from build123d import *

# Parameters (mm, degrees)
F0_R     = 5.25
F0_R_2   = 18.800913
F0_R_3   = 5.254085
F0_R_4   = 5.311104
F1_DEPTH = 10


with BuildPart() as f1:
    # F0 (on Front) → F1 (new body)
    with BuildSketch(Plane.XZ):
        with BuildLine():
            Line((195, 23.072333), (195, 73.480297))
            ThreePointArc((195, 73.480297), (193.122359, 78.251192), (188.496733, 80.46265))
            Line((188.496733, 80.46265), (185.082949, 80.705511))
            ThreePointArc((185.082949, 80.705511), (180.133201, 78.655259), (178.082949, 73.705511))
            Line((178.082949, 73.705511), (178.082949, 72.705511))
            ThreePointArc((178.082949, 72.705511), (176.032696, 67.755764), (171.082949, 65.705511))
            Line((171.082949, 65.705511), (110.082949, 65.705511))
            ThreePointArc((110.082949, 65.705511), (105.133201, 67.755764), (103.082949, 72.705511))
            Line((103.082949, 72.705511), (103.082949, 73.705511))
            ThreePointArc((103.082949, 73.705511), (101.032696, 78.655259), (96.082949, 80.705511))
            Line((96.082949, 80.705511), (93.082949, 80.705511))
            ThreePointArc((93.082949, 80.705511), (88.133201, 78.655259), (86.082949, 73.705511))
            Line((86.082949, 73.705511), (86.082949, 72.705511))
            ThreePointArc((86.082949, 72.705511), (84.032696, 67.755764), (79.082949, 65.705511))
            Line((79.082949, 65.705511), (18.082949, 65.705511))
            ThreePointArc((18.082949, 65.705511), (13.133201, 67.755764), (11.082949, 72.705511))
            Line((11.082949, 72.705511), (11.082949, 73.705511))
            ThreePointArc((11.082949, 73.705511), (9.032696, 78.655259), (4.082949, 80.705511))
            Line((4.082949, 80.705511), (1.082949, 80.705511))
            ThreePointArc((1.082949, 80.705511), (-3.866799, 78.655259), (-5.917051, 73.705511))
            Line((-5.917051, 73.705511), (-5.917051, 72.705511))
            ThreePointArc((-5.917051, 72.705511), (-7.967304, 67.755764), (-12.917051, 65.705511))
            Line((-12.917051, 65.705511), (-73.917051, 65.705511))
            ThreePointArc((-73.917051, 65.705511), (-78.866799, 67.755764), (-80.917051, 72.705511))
            Line((-80.917051, 72.705511), (-80.917051, 73.705511))
            ThreePointArc((-80.917051, 73.705511), (-82.967304, 78.655259), (-87.917051, 80.705511))
            Line((-87.917051, 80.705511), (-90.917051, 80.705511))
            ThreePointArc((-90.917051, 80.705511), (-95.866799, 78.655259), (-97.917051, 73.705511))
            Line((-97.917051, 73.705511), (-97.917051, 72.705511))
            ThreePointArc((-97.917051, 72.705511), (-99.967304, 67.755764), (-104.917051, 65.705511))
            Line((-104.917051, 65.705511), (-165.917051, 65.705511))
            ThreePointArc((-165.917051, 65.705511), (-170.866799, 67.755764), (-172.917051, 72.705511))
            Line((-172.917051, 72.705511), (-172.917051, 73.705511))
            ThreePointArc((-172.917051, 73.705511), (-174.967304, 78.655259), (-179.917051, 80.705511))
            Line((-179.917051, 80.705511), (-187.917051, 80.705511))
            ThreePointArc((-187.917051, 80.705511), (-191.62203, 79.64463), (-194.203996, 76.78355))
            ThreePointArc((-194.203996, 76.78355), (-194.606342, 74.960742), (-194.128551, 73.156241))
            Line((-194.128551, 73.156241), (-190.179633, 51.218559))
            ThreePointArc((-190.179633, 51.218559), (-190.114418, 50.911785), (-190.030097, 50.609704))
            Line((-190.030097, 50.609704), (-186.59138, 39.632266))
            ThreePointArc((-186.59138, 39.632266), (-186.208592, 38.609697), (-185.716602, 37.634957))
            Line((-185.716602, 37.634957), (-177.611824, 23.546821))
            ThreePointArc((-177.611824, 23.546821), (-176.740115, 22.270978), (-175.682257, 21.144661))
            Line((-175.682257, 21.144661), (-171.066362, 16.935058))
            ThreePointArc((-171.066362, 16.935058), (-169.380238, 14.933988), (-168.270966, 12.564006))
            Line((-168.270966, 12.564006), (-165.841167, 4.887599))
            ThreePointArc((-165.841167, 4.887599), (-163.303518, 1.352575), (-159.167506, 0))
            Line((-159.167506, 0), (-155, 0))
            Line((-155, 0), (-150.832494, 0))
            ThreePointArc((-150.832494, 0), (-146.696482, 1.352575), (-144.158833, 4.887599))
            Line((-144.158833, 4.887599), (-141.729034, 12.564006))
            ThreePointArc((-141.729034, 12.564006), (-140.619762, 14.933988), (-138.933638, 16.935058))
            Line((-138.933638, 16.935058), (-134.317743, 21.144661))
            ThreePointArc((-134.317743, 21.144661), (-133.259885, 22.270978), (-132.388176, 23.546821))
            Line((-132.388176, 23.546821), (-124.283398, 37.634957))
            Line((-124.283398, 37.634957), (-95.716602, 37.634957))
            Line((-95.716602, 37.634957), (-87.611824, 23.546821))
            ThreePointArc((-87.611824, 23.546821), (-86.740115, 22.270978), (-85.682257, 21.144661))
            Line((-85.682257, 21.144661), (-81.066362, 16.935058))
            ThreePointArc((-81.066362, 16.935058), (-79.380238, 14.933988), (-78.270966, 12.564006))
            Line((-78.270966, 12.564006), (-75.841167, 4.887599))
            ThreePointArc((-75.841167, 4.887599), (-73.303518, 1.352575), (-69.167506, 0))
            Line((-69.167506, 0), (-60.832494, 0))
            ThreePointArc((-60.832494, 0), (-56.696482, 1.352575), (-54.158833, 4.887599))
            Line((-54.158833, 4.887599), (-51.729034, 12.564006))
            ThreePointArc((-51.729034, 12.564006), (-50.619762, 14.933988), (-48.933638, 16.935058))
            Line((-48.933638, 16.935058), (-44.317743, 21.144661))
            ThreePointArc((-44.317743, 21.144661), (-43.259885, 22.270978), (-42.388176, 23.546821))
            Line((-42.388176, 23.546821), (-34.283398, 37.634957))
            Line((-34.283398, 37.634957), (-5.716602, 37.634957))
            Line((-5.716602, 37.634957), (0, 27.69807))
            Line((0, 27.69807), (2.388176, 23.546821))
            ThreePointArc((2.388176, 23.546821), (3.259885, 22.270978), (4.317743, 21.144661))
            Line((4.317743, 21.144661), (8.933638, 16.935058))
            ThreePointArc((8.933638, 16.935058), (10.619762, 14.933988), (11.729034, 12.564006))
            Line((11.729034, 12.564006), (14.158833, 4.887599))
            ThreePointArc((14.158833, 4.887599), (16.696482, 1.352575), (20.832494, 0))
            Line((20.832494, 0), (29.167506, 0))
            ThreePointArc((29.167506, 0), (33.303518, 1.352575), (35.841167, 4.887599))
            Line((35.841167, 4.887599), (38.270966, 12.564006))
            ThreePointArc((38.270966, 12.564006), (39.380238, 14.933988), (41.066362, 16.935058))
            Line((41.066362, 16.935058), (45.682257, 21.144661))
            ThreePointArc((45.682257, 21.144661), (46.740115, 22.270978), (47.611824, 23.546821))
            Line((47.611824, 23.546821), (55.716602, 37.634957))
            Line((55.716602, 37.634957), (84.283398, 37.634957))
            Line((84.283398, 37.634957), (92.388176, 23.546821))
            ThreePointArc((92.388176, 23.546821), (93.259885, 22.270978), (94.317743, 21.144661))
            Line((94.317743, 21.144661), (98.933638, 16.935058))
            ThreePointArc((98.933638, 16.935058), (100.619762, 14.933988), (101.729034, 12.564006))
            Line((101.729034, 12.564006), (104.158833, 4.887599))
            ThreePointArc((104.158833, 4.887599), (106.696482, 1.352575), (110.832494, 0))
            Line((110.832494, 0), (116.678365, 0))
            ThreePointArc((116.678365, 0), (121.628113, 2.050253), (123.678365, 7))
            Line((123.678365, 7), (123.678365, 9.434213))
            Line((123.678365, 9.434213), (125.800882, 14.62259))
            ThreePointArc((125.800882, 14.62259), (126.842165, 16.38046), (128.346681, 17.762781))
            Line((128.346681, 17.762781), (135.855722, 22.862975))
            ThreePointArc((135.855722, 22.862975), (137.704573, 23.750323), (139.732566, 24.055079))
            Line((139.732566, 24.055079), (173.859254, 24.055079))
            ThreePointArc((173.859254, 24.055079), (177.424201, 23.079292), (179.995255, 20.423979))
            Line((179.995255, 20.423979), (180.390863, 19.703433))
            ThreePointArc((180.390863, 19.703433), (182.961917, 17.048119), (186.526864, 16.072333))
            Line((186.526864, 16.072333), (188, 16.072333))
            ThreePointArc((188, 16.072333), (192.949747, 18.122585), (195, 23.072333))
        make_face()
        with Locations((-155, 9.734498)):
            Circle(F0_R, mode=Mode.SUBTRACT)
        with Locations((-65, 9.734498)):
            Circle(F0_R, mode=Mode.SUBTRACT)
        with Locations((-155, 39.055079)):
            Circle(F0_R_2, mode=Mode.SUBTRACT)
        with Locations((-65, 39.055079)):
            Circle(F0_R_2, mode=Mode.SUBTRACT)
        with Locations((25, 9.734498)):
            Circle(F0_R, mode=Mode.SUBTRACT)
        with Locations((115, 9.734498)):
            Circle(F0_R, mode=Mode.SUBTRACT)
        with Locations((25, 39.055079)):
            Circle(F0_R_2, mode=Mode.SUBTRACT)
        with Locations((186.789841, 24.055079)):
            Circle(F0_R, mode=Mode.SUBTRACT)
        with Locations((115, 39.055079)):
            Circle(F0_R_2, mode=Mode.SUBTRACT)
        with Locations((-183.994836, 73.705511)):
            Circle(F0_R_3, mode=Mode.SUBTRACT)
        with Locations((-89.581637, 73.705511)):
            Circle(F0_R_4, mode=Mode.SUBTRACT)
        with BuildLine():
            ThreePointArc((7.963389, 73.705511), (5.293816, 69.133433), (0, 69.211068))
            ThreePointArc((0, 69.211068), (-2.536611, 73.705511), (0, 78.199955))
            ThreePointArc((0, 78.199955), (5.293816, 78.277589), (7.963389, 73.705511))
        make_face(mode=Mode.SUBTRACT)
        with Locations((94.714896, 73.705511)):
            Circle(F0_R, mode=Mode.SUBTRACT)
        with Locations((186.789841, 73.705511)):
            Circle(F0_R, mode=Mode.SUBTRACT)
    extrude(amount=F1_DEPTH)


solid = f1.part
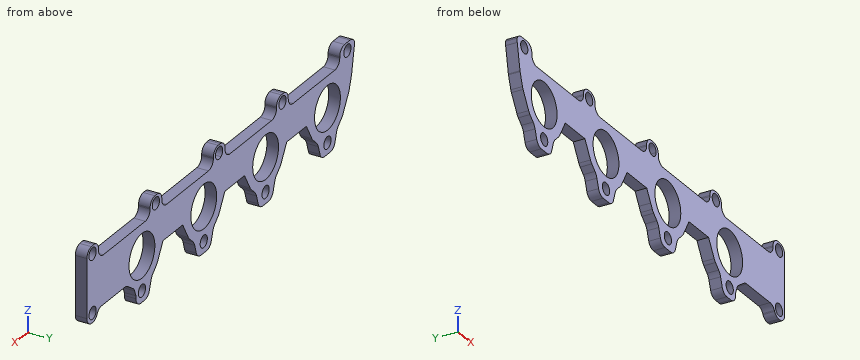
Can you work these out from the model? Positions are in its coordinate system, mm. Give positions to 0.01 mm unless a question says otherwise; leave off trailing zeros. Write each loop counter-clockwise with the first axis right and the second up, starting at its lowest first coordinate (ties: lowest second). Pieces come first, ordered by that corner, then holes. Notation, with made-up numbers: M 76.25,67 L 82.25,67 A16 ccw 82.25,97 Z; hole C 73,-25 d10. An arc over 180 degrees is marked long. Answer in a Markdown table with one row per item. Add a question column.
Item 1: Imagine slicing it at A-A, the plane x = -65. Write out the boundary of the cut face in (y, z).
Item 2: Please list where these lines run through material, in increasing order: L1, parallel to Z at x = 25, y = -3; L2, parallel to Z at x = -90, y = -9; L3, parallel to X at y = -8, z = 53.
Item 3: Imagine slicing it at B-B, the plane y = -3. State how many separate pieces and enclosed holes the cut face has, plus the area to 3 significant figures.
Item 4: For pin 1 Ø0.7 at (y, z) = (-4.5, 8) entering from +X; pin 2 Ø0.5 at (y, z) = (-6.5, 73.5) entering from -X; pin 3 Ø1.1 at (y, z) = (-5, 73.5) entering from -X, each with a flat end and sliding along its axis, tell me the tip position at first contact or that it passes through.
Evaluation:
| question | item | result |
|---|---|---|
| 1 | outline | M -10,0 L 0,0 L 0,4.48 L -10,4.48 Z; M -10,14.98 L 0,14.98 L 0,20.25 L -10,20.25 Z; M -10,57.86 L 0,57.86 L 0,65.71 L -10,65.71 Z |
| 2 | L1 | z = 0 to 4.48, 14.98 to 20.25, 57.86 to 65.71 |
| 2 | L2 | z = 27.7 to 68.41, 79 to 80.71 |
| 2 | L3 | x = -190.5 to -167.61, -142.39 to -77.61, -52.39 to 12.39, 37.61 to 102.39, 127.61 to 195 |
| 3 | separate pieces | 1 |
| 3 | enclosed holes | 14 |
| 3 | area | 13,200 mm² |
| 4 | pin 1 | stops at x = 123.68 |
| 4 | pin 2 | stops at x = -194.39 |
| 4 | pin 3 | stops at x = -194.48 |
